The listing builds one solid part. Answer for the finished solid, in the listing's coordinates (mm). A direction names the side the tool comes from. Coordinates: 2 decimals unless noted, no trailing zeros. Order: outer loops, then holes, each group sorted by start corner. A loop starts at its lowest first (then second) coordinate and runs counter-clockwise, first axis right, second up. Notation, with made-up numbers: (57.5, 67) -> (88.5, 67) arc R29 ccw to (88.5, 103) -> close; hole circle Ø9 at (79.25, 67.25). An arc over 180 degrees is marked (long way). Return JSON: item names as keys, results as strings.
```python
from build123d import *

# Parameters (mm, degrees)
SKETCH2_W                = 67.5
SKETCH2_H                = 67.5
SKETCH2_R                = 1.65
BOSS_EXTRUDE3_DEPTH      = 10
BOSS_EXTRUDE6_DEPTH      = 10
CUT_EXTRUDE2_DEPTH       = 10
CUT_EXTRUDE3_DEPTH       = 10
SKETCH13_W               = 20
SKETCH13_H               = 10
BOSS_EXTRUDE8_DEPTH      = 59.282032303
BOSS_EXTRUDE9_DEPTH      = 77.5
BOSS_EXTRUDE9_DEPTH_BACK = 77.5
SKETCH14_W               = 55
SKETCH14_H               = 52.5
SKETCH15_W               = 150
SKETCH15_H               = 50
CUT_EXTRUDE4_DEPTH       = 50
FILLET1_R                = 10


with BuildPart() as part:
    # Sketch2 → Boss-Extrude3 (new body)
    with BuildSketch(Plane(origin=(0, 0, 0), x_dir=(1, 0, 0), z_dir=(0, 1, 0))):
        Rectangle(SKETCH2_W, SKETCH2_H)
        with Locations(Location((-30, 0, 0), (0, 0, 270))):
            Circle(SKETCH2_R, mode=Mode.SUBTRACT)
        with Locations(Location((30, 0, 0), (0, 0, 270))):
            Circle(SKETCH2_R, mode=Mode.SUBTRACT)
        with Locations(Location((0, -30, 0), (0, 0, 270))):
            Circle(SKETCH2_R, mode=Mode.SUBTRACT)
    extrude(amount=BOSS_EXTRUDE3_DEPTH)


with BuildPart() as body_2:
    # Sketch5 → Boss-Extrude6 (new, symmetric)
    with BuildSketch(Plane(origin=(0, 0, 0), x_dir=(0.7071067811865476, 0, -0.7071067811865476), z_dir=(0.7071067811865476, 0, 0.7071067811865476))):
        Polygon((-37.72970773, 10), (-157.72970773, -59.282032303), (-140.409199654, -59.282032303), (-37.72970773, 0), align=None)
    boss_extrude6 = extrude(amount=BOSS_EXTRUDE6_DEPTH, both=True)


with BuildPart() as part_1:
    add(part.part)

    # Mirror3: Boss-Extrude6 across plane
    add(boss_extrude6.mirror(Plane(origin=(0, 0, 0), x_dir=(0, 0, 1), z_dir=(1, 0, 0))))

    # Sketch11 → Cut-Extrude2 (cut)
    with BuildSketch(Plane(origin=(9.731595226, 23.837442686, 9.731595226), x_dir=(0.9259415151999266, -0.2703581015304675, -0.2637021186227093), z_dir=(0.35355339059327223, 0.8660254037844399, 0.3535533905932725))):
        Polygon((6.552208132, -28.687416212), (23.376309745, -17.873092151), (23.376309745, -36.367082054), align=None)
    extrude(amount=CUT_EXTRUDE2_DEPTH, mode=Mode.SUBTRACT)

    # Sketch12 → Cut-Extrude3 (cut)
    with BuildSketch(Plane(origin=(-9.731595226, 23.837442686, 9.731595226), x_dir=(0.9259415151999266, 0.2703581015304675, 0.2637021186227093), z_dir=(-0.35355339059327223, 0.8660254037844399, 0.3535533905932725))):
        Polygon((-98.300144639, -134.433887296), (-81.476043026, -145.248211357), (-6.552208132, -28.687416212), (-23.376309745, -17.873092151), align=None)
    extrude(amount=CUT_EXTRUDE3_DEPTH, mode=Mode.SUBTRACT)

    # Sketch13 → Boss-Extrude8 (add)
    with BuildSketch(Plane.XZ):
        with Locations((0, -28.75)):
            Rectangle(SKETCH13_W, SKETCH13_H)
    extrude(amount=BOSS_EXTRUDE8_DEPTH)

    add(body_2.part)  # Boss-Extrude9 merges body 2
    # Sketch14 → Boss-Extrude9 (add, two sides: drawn at the far end of the back side and taken through both)
    with BuildSketch(Plane(origin=(0, 0, 0), x_dir=(0, 0, -1), z_dir=(1, 0, 0)).offset(-BOSS_EXTRUDE9_DEPTH_BACK)):
        with Locations((-107.465780691, -23.032032303)):
            Rectangle(SKETCH14_W, SKETCH14_H)
    extrude(amount=BOSS_EXTRUDE9_DEPTH + BOSS_EXTRUDE9_DEPTH_BACK)

    # Sketch15 → Cut-Extrude4 (cut)
    with BuildSketch(Plane(origin=(0, 3.217967697, 0), x_dir=(1, 0, 0), z_dir=(0, 1, 0))):
        with Locations((0, -107.465780691)):
            Rectangle(SKETCH15_W, SKETCH15_H)
    extrude(amount=-CUT_EXTRUDE4_DEPTH, mode=Mode.SUBTRACT)

    # Fillet1
    # the kernel refuses this fillet: 10 mm, written as the material it adds along each edge
    with BuildSketch(Plane(origin=(-19.607864376, 0, 33.75), x_dir=(-0.7071067811865471, 0, 0.7071067811865479), z_dir=(0, 1, 0))) as fillet1_piece_1_section:
        with BuildLine():
            CenterArc((FILLET1_R * 0.414213562373, FILLET1_R), FILLET1_R, 225, 45)
            Line((-FILLET1_R * 0.292893218813, FILLET1_R * 0.292893218813), (0, 0))
            Line((0, 0), (FILLET1_R * 0.414213562373, 0))
        make_face()
    fillet1_piece_1 = extrude(amount=10, mode=Mode.PRIVATE)
    fillet1_piece_1 = split(fillet1_piece_1, bisect_by=Plane(origin=(-17.351540007, 0.866448536, 33.883967569), z_dir=(0.3535533905932724, -0.8660254037844399, -0.3535533905932724)), keep=Keep.TOP, mode=Mode.PRIVATE)
    add(fillet1_piece_1)
    with BuildSketch(Plane(origin=(-19.607864376, -10.355339059, 33.75), x_dir=(-0.7071067811865475, 0, 0.7071067811865475), z_dir=(0, 1, 0))) as fillet1_piece_2_section:
        with BuildLine():
            CenterArc((FILLET1_R * 0.414213562373, FILLET1_R), FILLET1_R, 225, 45)
            Line((-FILLET1_R * 0.292893218813, FILLET1_R * 0.292893218813), (0, 0))
            Line((0, 0), (FILLET1_R * 0.414213562373, 0))
        make_face()
    fillet1_piece_2 = extrude(amount=20.355339059, mode=Mode.PRIVATE)
    fillet1_piece_2 = split(fillet1_piece_2, bisect_by=Plane(origin=(-21.014554375, -1.158148748, 35.180183481), z_dir=(-0.3535533905932724, 0.8660254037844399, 0.3535533905932724)), keep=Keep.TOP, mode=Mode.PRIVATE)
    fillet1_piece_2 = split(fillet1_piece_2, bisect_by=Plane(origin=(-21.217188194, 0, 35.382817301), z_dir=(0, -1, 0)), keep=Keep.TOP, mode=Mode.PRIVATE)
    add(fillet1_piece_2)
    with BuildSketch(Plane(origin=(-19.607864376, 0, 33.75), x_dir=(-0.7071067811865471, 0, 0.7071067811865479), z_dir=(0, 1, 0))) as fillet1_piece_3_section:
        with BuildLine():
            CenterArc((FILLET1_R * 0.414213562373, FILLET1_R), FILLET1_R, 225, 45)
            Line((-FILLET1_R * 0.292893218813, FILLET1_R * 0.292893218813), (0, 0))
            Line((0, 0), (FILLET1_R * 0.414213562373, 0))
        make_face()
    fillet1_piece_3 = extrude(amount=10, mode=Mode.PRIVATE)
    fillet1_piece_3 = split(fillet1_piece_3, bisect_by=Plane(origin=(-20.84268256, 8.638165162, 35.850982283), z_dir=(0.3535533905932724, -0.8660254037844399, -0.3535533905932724)), keep=Keep.TOP, mode=Mode.PRIVATE)
    fillet1_piece_3 = split(fillet1_piece_3, bisect_by=Plane(origin=(-17.780820381, 1.138165162, 32.789120105), z_dir=(-0.3535533905932724, 0.8660254037844399, 0.3535533905932724)), keep=Keep.TOP, mode=Mode.PRIVATE)
    add(fillet1_piece_3)
    with BuildSketch(Plane(origin=(33.75, -10.355339059, 19.607864376), x_dir=(0, 0, -1), z_dir=(0, 1, 0))) as fillet1_piece_4_section:
        with BuildLine():
            CenterArc((FILLET1_R * 0.414213562373, -FILLET1_R), FILLET1_R, 90, 45)
            Line((-FILLET1_R * 0.292893218813, -FILLET1_R * 0.292893218813), (0, 0))
            Line((0, 0), (FILLET1_R * 0.414213562373, 0))
        make_face()
    fillet1_piece_4 = extrude(amount=20.355339059, mode=Mode.PRIVATE)
    fillet1_piece_4 = split(fillet1_piece_4, bisect_by=Plane(origin=(35.382817302, 0, 21.217188197), z_dir=(0, -1, 0)), keep=Keep.TOP, mode=Mode.PRIVATE)
    fillet1_piece_4 = split(fillet1_piece_4, bisect_by=Plane(origin=(35.180183482, -1.15814875, 21.014554377), z_dir=(0.35355339059327234, 0.8660254037844399, 0.35355339059327234)), keep=Keep.TOP, mode=Mode.PRIVATE)
    add(fillet1_piece_4)
    with BuildSketch(Plane(origin=(33.75, 0, 19.607864376), x_dir=(0, 0, -1), z_dir=(0, 1, 0))) as fillet1_piece_5_section:
        with BuildLine():
            CenterArc((FILLET1_R * 0.414213562373, -FILLET1_R), FILLET1_R, 90, 45)
            Line((-FILLET1_R * 0.292893218813, -FILLET1_R * 0.292893218813), (0, 0))
            Line((0, 0), (FILLET1_R * 0.414213562373, 0))
        make_face()
    fillet1_piece_5 = extrude(amount=10, mode=Mode.PRIVATE)
    fillet1_piece_5 = split(fillet1_piece_5, bisect_by=Plane(origin=(33.883967571, 0.866448534, 17.351540009), z_dir=(-0.35355339059327234, -0.8660254037844399, -0.35355339059327234)), keep=Keep.TOP, mode=Mode.PRIVATE)
    add(fillet1_piece_5)
    with BuildSketch(Plane(origin=(33.75, 0, 19.607864376), x_dir=(0, 0, -1), z_dir=(0, 1, 0))) as fillet1_piece_6_section:
        with BuildLine():
            CenterArc((FILLET1_R * 0.414213562373, -FILLET1_R), FILLET1_R, 90, 45)
            Line((-FILLET1_R * 0.292893218813, -FILLET1_R * 0.292893218813), (0, 0))
            Line((0, 0), (FILLET1_R * 0.414213562373, 0))
        make_face()
    fillet1_piece_6 = extrude(amount=10, mode=Mode.PRIVATE)
    fillet1_piece_6 = split(fillet1_piece_6, bisect_by=Plane(origin=(35.850982284, 8.638165162, 20.842682559), z_dir=(-0.3535533905932724, -0.8660254037844399, -0.3535533905932724)), keep=Keep.TOP, mode=Mode.PRIVATE)
    fillet1_piece_6 = split(fillet1_piece_6, bisect_by=Plane(origin=(32.789120106, 1.138165162, 17.780820381), z_dir=(0.35355339059327234, 0.8660254037844399, 0.35355339059327234)), keep=Keep.TOP, mode=Mode.PRIVATE)
    add(fillet1_piece_6)
    with BuildSketch(Plane(origin=(-33.75, 0, 19.607864376), x_dir=(-0.7071067811865479, 0, 0.7071067811865471), z_dir=(0, 1, 0))) as fillet1_piece_7_section:
        with BuildLine():
            CenterArc((FILLET1_R * 0.414213562373, -FILLET1_R), FILLET1_R, 90, 45)
            Line((-FILLET1_R * 0.292893218813, -FILLET1_R * 0.292893218813), (0, 0))
            Line((0, 0), (FILLET1_R * 0.414213562373, 0))
        make_face()
    fillet1_piece_7 = extrude(amount=10, mode=Mode.PRIVATE)
    fillet1_piece_7 = split(fillet1_piece_7, bisect_by=Plane(origin=(-33.883967569, 0.866448536, 17.351540007), z_dir=(0.3535533905932724, -0.8660254037844399, -0.3535533905932724)), keep=Keep.TOP, mode=Mode.PRIVATE)
    add(fillet1_piece_7)
    with BuildSketch(Plane(origin=(-33.75, -10.355339059, 19.607864376), x_dir=(-0.7071067811865475, 0, 0.7071067811865475), z_dir=(0, 1, 0))) as fillet1_piece_8_section:
        with BuildLine():
            CenterArc((FILLET1_R * 0.414213562373, -FILLET1_R), FILLET1_R, 90, 45)
            Line((-FILLET1_R * 0.292893218813, -FILLET1_R * 0.292893218813), (0, 0))
            Line((0, 0), (FILLET1_R * 0.414213562373, 0))
        make_face()
    fillet1_piece_8 = extrude(amount=20.355339059, mode=Mode.PRIVATE)
    fillet1_piece_8 = split(fillet1_piece_8, bisect_by=Plane(origin=(-35.180183481, -1.158148748, 21.014554375), z_dir=(-0.3535533905932724, 0.8660254037844399, 0.3535533905932724)), keep=Keep.TOP, mode=Mode.PRIVATE)
    fillet1_piece_8 = split(fillet1_piece_8, bisect_by=Plane(origin=(-35.382817301, 0, 21.217188194), z_dir=(0, -1, 0)), keep=Keep.TOP, mode=Mode.PRIVATE)
    add(fillet1_piece_8)
    with BuildSketch(Plane(origin=(-33.75, 0, 19.607864376), x_dir=(-0.7071067811865479, 0, 0.7071067811865471), z_dir=(0, 1, 0))) as fillet1_piece_9_section:
        with BuildLine():
            CenterArc((FILLET1_R * 0.414213562373, -FILLET1_R), FILLET1_R, 90, 45)
            Line((-FILLET1_R * 0.292893218813, -FILLET1_R * 0.292893218813), (0, 0))
            Line((0, 0), (FILLET1_R * 0.414213562373, 0))
        make_face()
    fillet1_piece_9 = extrude(amount=10, mode=Mode.PRIVATE)
    fillet1_piece_9 = split(fillet1_piece_9, bisect_by=Plane(origin=(-35.850982283, 8.638165162, 20.84268256), z_dir=(0.3535533905932724, -0.8660254037844399, -0.3535533905932724)), keep=Keep.TOP, mode=Mode.PRIVATE)
    fillet1_piece_9 = split(fillet1_piece_9, bisect_by=Plane(origin=(-32.789120105, 1.138165162, 17.780820381), z_dir=(-0.3535533905932724, 0.8660254037844399, 0.3535533905932724)), keep=Keep.TOP, mode=Mode.PRIVATE)
    add(fillet1_piece_9)
    with BuildSketch(Plane(origin=(19.607864376, -10.355339059, 33.75), x_dir=(-1, 0, 0), z_dir=(0, 1, 0))) as fillet1_piece_10_section:
        with BuildLine():
            CenterArc((FILLET1_R * 0.414213562373, FILLET1_R), FILLET1_R, 225, 45)
            Line((-FILLET1_R * 0.292893218813, FILLET1_R * 0.292893218813), (0, 0))
            Line((0, 0), (FILLET1_R * 0.414213562373, 0))
        make_face()
    fillet1_piece_10 = extrude(amount=20.355339059, mode=Mode.PRIVATE)
    fillet1_piece_10 = split(fillet1_piece_10, bisect_by=Plane(origin=(21.217188197, 0, 35.382817302), z_dir=(0, -1, 0)), keep=Keep.TOP, mode=Mode.PRIVATE)
    fillet1_piece_10 = split(fillet1_piece_10, bisect_by=Plane(origin=(21.014554377, -1.15814875, 35.180183482), z_dir=(0.35355339059327234, 0.8660254037844399, 0.35355339059327234)), keep=Keep.TOP, mode=Mode.PRIVATE)
    add(fillet1_piece_10)
    with BuildSketch(Plane(origin=(19.607864376, 0, 33.75), x_dir=(-1, 0, 0), z_dir=(0, 1, 0))) as fillet1_piece_11_section:
        with BuildLine():
            CenterArc((FILLET1_R * 0.414213562373, FILLET1_R), FILLET1_R, 225, 45)
            Line((-FILLET1_R * 0.292893218813, FILLET1_R * 0.292893218813), (0, 0))
            Line((0, 0), (FILLET1_R * 0.414213562373, 0))
        make_face()
    fillet1_piece_11 = extrude(amount=10, mode=Mode.PRIVATE)
    fillet1_piece_11 = split(fillet1_piece_11, bisect_by=Plane(origin=(17.351540009, 0.866448534, 33.883967571), z_dir=(-0.35355339059327234, -0.8660254037844399, -0.35355339059327234)), keep=Keep.TOP, mode=Mode.PRIVATE)
    add(fillet1_piece_11)
    with BuildSketch(Plane(origin=(19.607864376, 0, 33.75), x_dir=(-1, 0, 0), z_dir=(0, 1, 0))) as fillet1_piece_12_section:
        with BuildLine():
            CenterArc((FILLET1_R * 0.414213562373, FILLET1_R), FILLET1_R, 225, 45)
            Line((-FILLET1_R * 0.292893218813, FILLET1_R * 0.292893218813), (0, 0))
            Line((0, 0), (FILLET1_R * 0.414213562373, 0))
        make_face()
    fillet1_piece_12 = extrude(amount=10, mode=Mode.PRIVATE)
    fillet1_piece_12 = split(fillet1_piece_12, bisect_by=Plane(origin=(20.842682559, 8.638165162, 35.850982284), z_dir=(-0.3535533905932724, -0.8660254037844399, -0.3535533905932724)), keep=Keep.TOP, mode=Mode.PRIVATE)
    fillet1_piece_12 = split(fillet1_piece_12, bisect_by=Plane(origin=(17.780820381, 1.138165162, 32.789120106), z_dir=(0.35355339059327234, 0.8660254037844399, 0.35355339059327234)), keep=Keep.TOP, mode=Mode.PRIVATE)
    add(fillet1_piece_12)


solid = part_1.part
```
Item 1: Find the intervals of material crossed by probe 1 along X at (y, z) = (6.5, 0); probe 2 along X at (y, z) = (-24, 111.5); probe 3 along Z at (x, y) = (-4, -8), in increasing order.
Answer list:
{"probe 1": "-33.75 to -31.65, -28.35 to 28.35, 31.65 to 33.75", "probe 2": "-77.5 to -75, 75 to 77.5", "probe 3": "-33.75 to -23.75, 79.97 to 82.47, 132.47 to 134.97"}
Item 2: The part is cut by section D-D on x = 25. Determine the outline of the cut face in (y, z).
Answer list:
{"outline": "(-49.28, 79.97) -> (3.22, 79.97) -> (3.22, 82.47) -> (-46.78, 82.47) -> (-46.78, 132.47) -> (3.22, 132.47) -> (3.22, 134.97) -> (-49.28, 134.97) -> close; (-4.4, 39.14) -> (0, 28.36) -> (0, -33.75) -> (10, -33.75) -> (10, 28.36) -> (5.6, 39.14) -> close"}
Item 3: The part is cut by section B-B on x = -57. Determine the outline of the cut face in (y, z), plus the area to 3 significant figures.
Answer list:
{"outline": "(-49.28, 79.97) -> (3.22, 79.97) -> (3.22, 82.47) -> (-46.78, 82.47) -> (-46.78, 132.47) -> (3.22, 132.47) -> (3.22, 134.97) -> (-49.28, 134.97) -> close; (-30.53, 71.14) -> (-18.98, 42.86) -> (-8.98, 42.86) -> (-20.53, 71.14) -> close", "area": "670 mm2"}
Item 4: The part is cut by section A-A on y = -10. Determine the outline of the cut face in (x, z).
Answer list:
{"outline": "(-77.5, 79.97) -> (77.5, 79.97) -> (77.5, 134.97) -> (-77.5, 134.97) -> close; (-58.24, 44.1) -> (-46, 31.86) -> (-31.86, 46) -> (-44.1, 58.24) -> close; (-10, -33.75) -> (10, -33.75) -> (10, -23.75) -> (-10, -23.75) -> close; (31.86, 46) -> (46, 31.86) -> (58.24, 44.1) -> (44.1, 58.24) -> close; hole (-75, 82.47) -> (75, 82.47) -> (75, 132.47) -> (-75, 132.47) -> close"}
Item 5: Determine the mould class of faces 4 (the flat face through (-1, -49.282, 108)), 5 (the flat face through (74.8, -30.64, 60.66)), 6 (the flat face through (0, 5, 33.75)) for opening direction Z: pulls with the +Z half, pulls with the -Z half, needs draft (parallel to the pull), parting line crosses it, or undercut.
Answer list:
{"face 4": "needs draft", "face 5": "pulls with the -Z half", "face 6": "undercut"}
Item 6: Which of the six approach directions +Z, -Z, +X, -X, +Y, -Y give full straight-line access (tool end or side, diameter ignored) to faces 1 (the flat face through (88.05, -49.85, 102.19)), 2 (the flat face through (-10, -29, -29)), 3 (the flat face through (-1, -21, 82.466))?
Answer list:
{"face 1": "+Z, +Y, -Y", "face 2": "-Z, -X, -Y", "face 3": "+Y"}
Item 7: Flat-ended cylindrical pins translate along their axes: pin 1 (8 mm diameter, centred on x = 54, y = -36, fed in from -Z); pin 2 (25 mm diameter, centred on x = -22, z = 103.5, fed in from +Y); pin 3 (3 mm diameter, centred on x = -30, z = 0, fed in from +Y); pin 4 (5 mm diameter, centred on x = -68.5, z = 76, fed in from -Y). Find the tip coordinate at first contact, or state that the pin passes through.
Answer list:
{"pin 1": "z = 79.97", "pin 2": "y = -46.78", "pin 3": "through", "pin 4": "y = -38.65"}
Item 8: The part is cut by section C-C on y = -52. Determine the outline of the cut face in (x, z).
Answer list:
{"outline": "(-109.68, 95.54) -> (-97.44, 83.29) -> (-83.29, 97.44) -> (-95.54, 109.68) -> close; (-10, -33.75) -> (10, -33.75) -> (10, -23.75) -> (-10, -23.75) -> close; (83.29, 97.44) -> (97.44, 83.29) -> (109.68, 95.54) -> (95.54, 109.68) -> close"}
